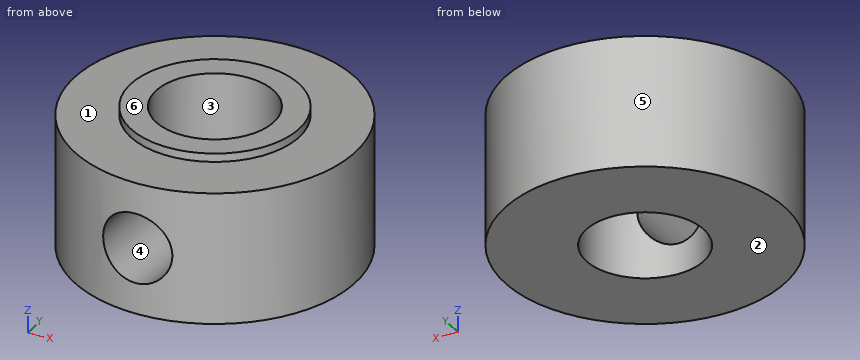
```python
from build123d import *

# Parameters (mm, degrees)
ESQUISSE1_R             = 5
BOSS_EXTRU_1_DEPTH      = 4.7
ESQUISSE2_R             = 3
BOSS_EXTRU_3_DEPTH      = 0.3
ESQUISSE3_R             = 2.1
ENL_V_MAT_EXTRU_1_DEPTH = 9.660254038
ESQUISSE4_R             = 1.25
ENL_V_MAT_EXTRU_2_DEPTH = 9.660254038


with BuildPart() as part:
    # Esquisse1 → Boss.-Extru.1 (new body)
    with BuildSketch(Plane.XY):
        Circle(ESQUISSE1_R)
    extrude(amount=BOSS_EXTRU_1_DEPTH)

    # Esquisse2 → Boss.-Extru.3 (add)
    with BuildSketch(Plane.XY.offset(4.7)):
        Circle(ESQUISSE2_R)
    extrude(amount=BOSS_EXTRU_3_DEPTH)

    # Esquisse3 → Enlèv. mat.-Extru.1 (cut, through all)
    with BuildSketch(Plane.XY.offset(5)):
        Circle(ESQUISSE3_R)
    extrude(amount=-ENL_V_MAT_EXTRU_1_DEPTH, mode=Mode.SUBTRACT)

    # Esquisse4 → Enlèv. mat.-Extru.2 (cut, through all)
    with BuildSketch(Plane(origin=(0, 0, 0), x_dir=(1, 0, 0), z_dir=(0, 1, 0))):
        with Locations(Location((0, -2.35, 0), (0, 0, 270))):
            Circle(ESQUISSE4_R)
    extrude(amount=-ENL_V_MAT_EXTRU_2_DEPTH, mode=Mode.SUBTRACT)


solid = part.part
```
Build history of the part. All positions in model axes, mm. Face numbers are marked on the shaded views. A direction names the side the tool comes from. Round coordinates to 2 decimals unless told otherwise and drop trailing zeros. Write each loop counter-clockwise with the first axis right and the second up, starting at its lowest first coordinate (ties: lowest second). Pieces come first, ordered by that corner, then holes. Notation, with made-up numbers: (82.25, 10.5) - (137.25, 10.5) arc R14 ccw to (137.25, 14.5) - close; hole circle Ø7 at (50.5, 28). An arc over 180 degrees is marked (long way). Write each question's results on one line, items separated by ' | '. Start each with the question number.
Item 1: Saw through at C-C (y = -3.5). Write the cut outline in (x, z).
Item 2: Mould opens along X. For the marked faces 3, 4, 5 and 6 say: pulls with the +X half, pulls with the -X half, needs draft (parallel to the pull), parting line crosses it, or undercut.
Item 3: Saw through at D-D (x = 4). Write the cut outline in (y, z).
Item 4: Saw through at B-B (x = 0). Write the cut outline in (y, z).
Item 5: Wall check: L1, parallel to Z at x = 3.5, y = -0.25; L2, parallel to Y at x = 0, z = 1.8; L3, parallel to Z at x = 0, y = -2.8. Give the ranges that are in metal, low to high. Write a range as [from, to].
Item 6: Which spindle directions (+Z, -Z, +X, -X, +Y, -Y) get a long thin tool onto all of the face, cutting with end or side? Do the marked faces 1 and 2. Say none if no direction does.
Item 7: Drop flat-ended pins along their axis: P1, Ø1, axis at x = -3, y = 2, coming from the +Z side; P2, Ø2, axis at x = 0, z = 2.35, coming from the -Y side; P3, Ø1, axis at x = 2, z = 3, coming from the -Y side. Give the stop position or say it passes through.
Item 8: Saw through at A-A (y = 0). Write the cut outline in (x, z).
Results are:
1) outline: (-3.57, 0) - (3.57, 0) - (3.57, 4.7) - (-3.57, 4.7) - close; hole circle Ø2.5 at (0, 2.35)
2) face 3: undercut | face 4: undercut | face 5: parting line crosses it | face 6: needs draft
3) outline: (-3, 0) - (3, 0) - (3, 4.7) - (-3, 4.7) - close
4) outline: (-5, 0) - (-2.1, 0) - (-2.1, 1.1) - (-5, 1.1) - close; (-5, 3.6) - (-2.1, 3.6) - (-2.1, 5) - (-3, 5) - (-3, 4.7) - (-5, 4.7) - close; (2.1, 0) - (5, 0) - (5, 4.7) - (3, 4.7) - (3, 5) - (2.1, 5) - close
5) L1: z = [0, 4.7] | L2: y = [2.1, 5] | L3: z = [0, 1.1], [3.6, 5]
6) face 1: +Z | face 2: -Z, +X, -X, +Y, -Y
7) P1: stops at z = 4.7 | P2: stops at y = 1.85 | P3: stops at y = -4.77
8) outline: (-5, 0) - (-2.1, 0) - (-2.1, 5) - (-3, 5) - (-3, 4.7) - (-5, 4.7) - close; (2.1, 0) - (5, 0) - (5, 4.7) - (3, 4.7) - (3, 5) - (2.1, 5) - close
